Can you work these out from the model? Positions are in its coordinate system, mm. Face numbers are marked on the shaded views. A direction names the side the tool comes from. Give positions to 0.01 mm unless a question says otherwise; leave off trailing zeros. Loops run counter-clockwise (first coordinate to the right, second up) from the corner with the lowest first, then second, coordinate; pieces in that order, holes last. Notation, with made-up numbers: (6.25, 82.5) - (31.25, 82.5) arc R22 cw to (31.25, 91.5) - close; hole circle Ø1 at (43.25, 7.5). An arc over 180 degrees is marked (long way). Answer as a JSON object with one key per item and string values. Group by question number.
Item 1: Will these pins go through, and if not, where does the flat tip stop? pin 1 (19.5 mm diameter, centred on x = -18, z = 31, fed in from -Y); pin 2 (6 mm diameter, centred on y = 21, z = 26.5, fed in from -X); pin 3 (15 mm diameter, centred on x = -5, z = 14, fed in from +Y); pin 4 (2 mm diameter, centred on y = 27.5, z = 12.5, fed in from +X).
Item 2: Suppose I cut it at D-D on y = 15.5. Write out the boundary of the cut face in (x, z).
Item 3: Which directions (+Z, -Z, +X, -X, +Y, -Y) give clear straight access to the entire face, cutting with the end or side of a thin tool? Please do the marked faces 1, 2 and 3.
Item 4: Please list where these lines run through material, in increasing order: L1, parallel to Z at x = -23, y = 26; L2, parallel to Y at x = -22, z = 36; L3, parallel to X at y = 0.5, z = 35.5.
Item 5: Suppose I cut it at C-C on x = -4.5. Write out the boundary of the cut face in (y, z), and give its area (3 significant figures).
from build123d import *

# Parameters (mm, degrees)
F1_DEPTH = 42
F2_R     = 1.49999
F4_D     = 2.2606
F4_DEPTH = 18.57375
F4_TIP   = 0.6791527577


# Not quite as in the source:
# - a fillet or chamfer is up to 0.001 mm smaller than in the source, because OpenCascade refuses the exact size


with BuildPart() as f1:
    # F0 (on Top) → F1 (new body)
    with BuildSketch(Plane.XY):
        with BuildLine():
            ThreePointArc((0, 19), (17.5537111177, 7.2709852149), (13.4350288425, -13.4350288425))
            Line((13.4350288425, -13.4350288425), (15.5563491861, -15.5563491861))
            ThreePointArc((15.5563491861, -15.5563491861), (20.8531990078, 7.0102846689), (3, 21.7944947177))
            Line((3, 21.7944947177), (3, 24))
            Line((3, 24), (-19, 24))
            Line((-19, 24), (-19, 31))
            Line((-19, 31), (-26, 31))
            Line((-26, 31), (-26, 21))
            Line((-26, 21), (0, 21))
            Line((0, 21), (0, 19))
        make_face()
    extrude(amount=F1_DEPTH)

    # F2 (radius 1.5 in the source; OpenCascade refuses exactly that, so slightly less here)
    f2_edges = [f1.edges().sort_by_distance(p)[0] for p in [
        (13.435029, -13.435029, 21),
        (15.556349, -15.556349, 21),
        (-26, 21, 21),
        (3, 24, 21),
        (-19, 24, 21),
        (-19, 31, 21),
    ]]
    fillet(f2_edges, radius=F2_R)

    # F4
    with Locations(Plane(origin=(-26, 0, 0), x_dir=(0, -1, 0), z_dir=(-1, 0, 0))):
        with Locations((-26, 36), (-26, 6)):
            Hole(F4_D / 2, depth=F4_DEPTH)
            with Locations((0, 0, -(F4_DEPTH + F4_TIP / 2))):  # 118° drill point
                Cone(0, F4_D / 2, F4_TIP, mode=Mode.SUBTRACT)


solid = f1.part
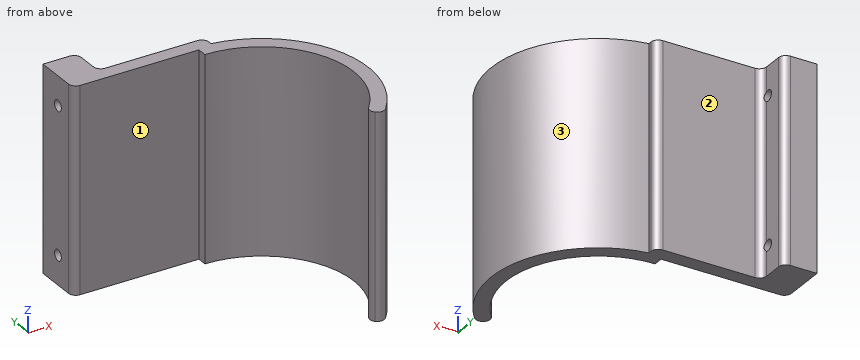
Worked out:
{
 "1": {"pin 1": "stops at y = 21", "pin 2": "stops at x = -26", "pin 3": "stops at y = 24", "pin 4": "stops at x = -19"},
 "2": {"outline": "(10.99, 0) - (15.61, 0) - (15.61, 42) - (10.99, 42) - close"},
 "3": {"face 1": "+Z, -Z, -X, -Y", "face 2": "+Z, -Z, +X, +Y", "face 3": "+Z, -Z, +X"},
 "4": {"L1": "z = 0 to 4.87, 7.13 to 34.87, 37.13 to 42", "L2": "y = 21 to 24.87, 27.13 to 31", "L3": "x = 18.99 to 21.99"},
 "5": {"outline": "(21, 0) - (24, 0) - (24, 42) - (21, 42) - close", "area": "126 mm2"}
}
